Build history of the part. All positions in model axes, mm. Face numbers are marked on the shaded views. A direction names the side the tool comes from. Round coordinates to 2 decimals unless told otherwise and drop trailing zeros. Write each loop counter-clockwise with the first axis right and the second up, starting at its lowest first coordinate (ties: lowest second). Pieces come first, ordered by that corner, then holes. Notation, with made-up numbers: (-24.5, 33.5) - (19.5, 33.5) arc R35 ccw to (19.5, 66.5) - close; hole circle Ø4 at (46, -5.5). An arc over 180 degrees is marked (long way). One line per question, with ' | ' between items.
from build123d import *

# Parameters (mm, degrees)
F0_R           = 19.05
F1_DEPTH       = 5.334
F2_R           = 9.398
F3_DEPTH       = 1.016
F4_R           = 9.525
F5_DEPTH       = 28.575
F6_W           = 12.7
F6_H           = 7.9248
F7_DEPTH       = 31.75
F9_D           = 12.7
F9_DEPTH       = 28.575
F9_CSINK_D     = 13.97
F9_CSINK_ANGLE = 90
F9_TIP         = 3.8154649308
F10_SIZE       = 0.762
F12_D          = 2.3876
F14_D          = 2.4892
F14_DEPTH      = 14.732
F14_TIP        = 0.7478311264
F16_D          = 3.175
F16_DEPTH      = 9.525
F16_TIP        = 0.9538662327
F18_D          = 4.3688
F18_DEPTH      = 1.905
F18_START      = 32.1342766
F18_TIP        = 1.3125199362
F20_DEPTH      = 3.81
F21_R          = 1.5748
F22_SIZE       = 0.762


# Not quite as in the source:
# - a length typed as a fraction of an inch, garbled in the dataset ("3 / 203.2 mm" for 3/8 in), is restored


with BuildPart() as f1:
    # F0 (on Top) → F1 (new body)
    with BuildSketch(Plane.XY):
        Circle(F0_R)
    extrude(amount=F1_DEPTH)

    # F2 (on face) → F3 (join)
    with BuildSketch(Plane.XY.offset(5.334)):
        Circle(F2_R)
    extrude(amount=F3_DEPTH)

    # F4 (on face) → F5 (join)
    with BuildSketch(Plane(origin=(0, 0, 0), x_dir=(1, 0, 0), z_dir=(0, 0, -1))):
        Circle(F4_R)
    extrude(amount=F5_DEPTH)

    # F6 (on face) → F7 (join)
    with BuildSketch(Plane(origin=(0, 0, -28.575), x_dir=(1, 0, 0), z_dir=(0, 0, -1))):
        Rectangle(F6_W, F6_H)
    extrude(amount=F7_DEPTH)

    # F9
    with Locations(Plane.XY.offset(6.35)):
        with Locations((0, 0)):
            CounterSinkHole(F9_D / 2, F9_CSINK_D / 2, depth=F9_DEPTH, counter_sink_angle=F9_CSINK_ANGLE)
            with Locations((0, 0, -(F9_DEPTH + F9_TIP / 2))):  # 118° drill point
                Cone(0, F9_D / 2, F9_TIP, mode=Mode.SUBTRACT)

    # F10
    f10_edges = [f1.edges().sort_by_distance(p)[0] for p in [
        (-9.525, 0, -28.575),
        (-19.05, 0, 0),
        (-19.05, 0, 5.334),
    ]]
    chamfer(f10_edges, length=F10_SIZE)

    # F12 (through all)
    with Locations(Plane(origin=(0, 0, -60.325), x_dir=(1, 0, 0), z_dir=(0, 0, -1))):
        with Locations((2.4892, -0.7874), (-2.4892, -0.7874)):
            Hole(F12_D / 2)

    # F14
    with Locations(Plane(origin=(0, 0, -60.325), x_dir=(1, 0, 0), z_dir=(0, 0, -1))):
        with Locations((2.4892, -0.7874), (-2.4892, -0.7874)):
            Hole(F14_D / 2, depth=F14_DEPTH)
            with Locations((0, 0, -(F14_DEPTH + F14_TIP / 2))):  # 118° drill point
                Cone(0, F14_D / 2, F14_TIP, mode=Mode.SUBTRACT)

    # F16
    with Locations(Plane(origin=(0, 0, -60.325), x_dir=(1, 0, 0), z_dir=(0, 0, -1))):
        with Locations((2.4892, -0.7874), (-2.4892, -0.7874)):
            Hole(F16_D / 2, depth=F16_DEPTH)
            with Locations((0, 0, -(F16_DEPTH + F16_TIP / 2))):  # 118° drill point
                Cone(0, F16_D / 2, F16_TIP, mode=Mode.SUBTRACT)

    # F18
    # its depths count from where the whole tool has entered the part; down to there all is cleared
    with Locations(Plane.XY.offset(6.35)):
        with Locations((2.4892, 0.7874), (-2.4892, 0.7874)):
            Hole(F18_D / 2, depth=F18_START)
    with Locations(Plane.XY.offset(6.35).offset(-F18_START)):
        with Locations((2.4892, 0.7874), (-2.4892, 0.7874)):
            Hole(F18_D / 2, depth=F18_DEPTH)
            with Locations((0, 0, -(F18_DEPTH + F18_TIP / 2))):  # 118° drill point
                Cone(0, F18_D / 2, F18_TIP, mode=Mode.SUBTRACT)

    # F19 (on face) → F20 (cut)
    with BuildSketch(Plane.XY.offset(5.334)):
        with BuildLine():
            ThreePointArc((15.875, 1.5875), (14.7524679849, 1.1225320151), (14.2875, 0))
            ThreePointArc((14.2875, 0), (14.7524679849, -1.1225320151), (15.875, -1.5875))
            ThreePointArc((15.875, -1.5875), (16.9975320151, -1.1225320151), (17.4625, 0))
            ThreePointArc((17.4625, 0), (16.9975320151, 1.1225320151), (15.875, 1.5875))
        make_face()
        with BuildLine():
            ThreePointArc((12.7, -1.5875), (13.8225320151, -1.1225320151), (14.2875, 0))
            ThreePointArc((14.2875, 0), (13.8225320151, 1.1225320151), (12.7, 1.5875))
            Line((12.7, 1.5875), (12.7, -1.5875))
        make_face()
        with BuildLine():
            ThreePointArc((12.7, 1.5875), (13.8225320151, 1.1225320151), (14.2875, 0))
            ThreePointArc((14.2875, 0), (14.7524679849, 1.1225320151), (15.875, 1.5875))
            Line((15.875, 1.5875), (12.7, 1.5875))
        make_face()
        with BuildLine():
            Line((12.7, -1.5875), (12.7, 1.5875))
            ThreePointArc((12.7, 1.5875), (11.1125, 0), (12.7, -1.5875))
        make_face()
        with BuildLine():
            ThreePointArc((15.875, -1.5875), (14.7524679849, -1.1225320151), (14.2875, 0))
            ThreePointArc((14.2875, 0), (13.8225320151, -1.1225320151), (12.7, -1.5875))
            Line((12.7, -1.5875), (15.875, -1.5875))
        make_face()
        with BuildLine():
            ThreePointArc((-12.7, -1.5875), (-11.5774679849, -1.1225320151), (-11.1125, 0))
            ThreePointArc((-11.1125, 0), (-11.5774679849, 1.1225320151), (-12.7, 1.5875))
            ThreePointArc((-12.7, 1.5875), (-13.8225320151, 1.1225320151), (-14.2875, 0))
            ThreePointArc((-14.2875, 0), (-13.8225320151, -1.1225320151), (-12.7, -1.5875))
        make_face()
        with BuildLine():
            Line((-15.875, -1.5875), (-12.7, -1.5875))
            ThreePointArc((-12.7, -1.5875), (-13.8225320151, -1.1225320151), (-14.2875, 0))
            ThreePointArc((-14.2875, 0), (-14.7524679849, -1.1225320151), (-15.875, -1.5875))
        make_face()
        with BuildLine():
            ThreePointArc((-14.2875, 0), (-13.8225320151, 1.1225320151), (-12.7, 1.5875))
            Line((-12.7, 1.5875), (-15.875, 1.5875))
            ThreePointArc((-15.875, 1.5875), (-14.7524679849, 1.1225320151), (-14.2875, 0))
        make_face()
        with BuildLine():
            ThreePointArc((-15.875, -1.5875), (-14.7524679849, -1.1225320151), (-14.2875, 0))
            ThreePointArc((-14.2875, 0), (-14.7524679849, 1.1225320151), (-15.875, 1.5875))
            ThreePointArc((-15.875, 1.5875), (-17.4625, 0), (-15.875, -1.5875))
        make_face()
    extrude(amount=-F20_DEPTH, mode=Mode.SUBTRACT)

    # F21
    f21_edges = [f1.edges().sort_by_distance(p)[0] for p in [
        (6.35, 3.9624, -44.45),
        (6.35, -3.9624, -44.45),
        (-6.35, -3.9624, -44.45),
        (-6.35, 3.9624, -44.45),
    ]]
    fillet(f21_edges, radius=F21_R)

    # F22
    f22_edges = [f1.edges().sort_by_distance(p)[0] for p in [
        (6.35, 0, -60.325),
        (5.888752, -3.501152, -60.325),
        (0, -3.9624, -60.325),
        (-6.35, 0, -60.325),
        (-5.888752, -3.501152, -60.325),
        (0, 3.9624, -60.325),
        (5.888752, 3.501152, -60.325),
    ]]
    chamfer(f22_edges, length=F22_SIZE)


solid = f1.part
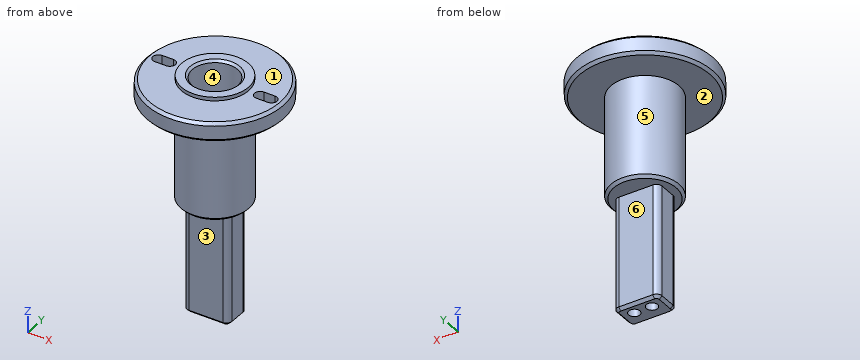
Q1. Drill centre lines: L1, parallel to X at y = 0, z = -5.5 (3 decimals); L2, parallel to X at y = 1.5, z = -35.5; L3, parallel to Y at x = 1.5, z = -52.5. Where is each one in solid material? Low to high. Write a range as from..to.
Found:
L1: -9.525..-6.35, 6.35..9.525 | L2: -6.35..-3.45, -1.53..1.53, 3.45..6.35 | L3: -3.96..-0.45, 2.03..3.96
Q2. Which spindle directions (+Z, -Z, +X, -X, +Y, -Y) get a long thin tool onto all of the face, cutting with end or side? Do the marked faces 1, 2 and 3. Say none if no direction does.
Found:
face 1: +Z | face 2: -Z | face 3: -Z, +X, -X, -Y
Q3. Saw through at B-B, the plane z = -5. List the corners of the cut face in (x, y) (3 decimals), then the cut area to 3 significant figures.
Found:
outline: circle Ø19.05 at (0, 0); hole circle Ø12.7 at (0, 0) | area: 158 mm^2
Q4. Pull direction X, two halves, no side cores. Call the marked faces 4, 5 and 6: +X half, -X half, draft (parallel to the pull), parting line (faces both ways), or undercut.
Found:
face 4: undercut | face 5: parting line | face 6: draft
Q5. Saw through at A-A, the plane z = -36. List the corners of the cut face in (x, y), then the cut area to 3 significant figures.
Found:
outline: (-6.35, -2.39) arc R1.57 ccw to (-4.78, -3.96) - (4.78, -3.96) arc R1.57 ccw to (6.35, -2.39) - (6.35, 2.39) arc R1.57 ccw to (4.78, 3.96) - (-4.78, 3.96) arc R1.57 ccw to (-6.35, 2.39) - close; hole circle Ø2.39 at (-2.49, 0.79); hole circle Ø2.39 at (2.49, 0.79) | area: 89.6 mm^2
Q6. Drop flat-ended pins along their axis: pin 1 (10 mm diameter, centred on x = 13.5, z = -7, fed in from -Y); pin 2 (7.5 mm diameter, centred on x = 1.5, z = -39.5, fed in from +Y); pin 3 (1 mm diameter, centred on x = 13, y = 0.5, fed in from +Z). Give the stop position or say it passes through.
Found:
pin 1: y = -4.3 | pin 2: y = 3.96 | pin 3: z = 1.52
